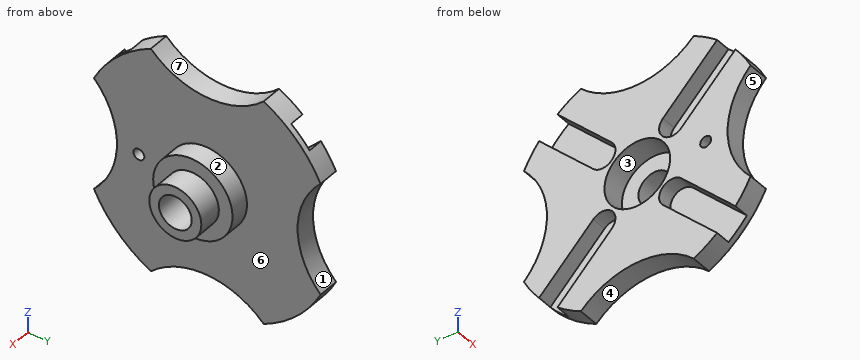
from build123d import *

# Parameters (mm, degrees)
ESQUISSE2_R             = 59
ENL_V_MAT_EXTRU_1_DEPTH = 139.666866987
ENL_V_START             = -11
ENL_V_MAT_EXTRU_2_DEPTH = 11
ESQUISSE4_R             = 4
ENL_V_MAT_EXTRU_3_DEPTH = 126.809424138


with BuildPart() as part:
    # Esquisse1 → Base-Révolution (revolve)
    with BuildSketch(Plane.XY, mode=Mode.PRIVATE) as base_r_volution_sk:
        Polygon((0, 24), (0, 92.5), (15, 92.5), (15, 29), (29, 29), (29, 19), (46, 19), (46, 12), (17, 12), (17, 24), align=None)
    revolve(base_r_volution_sk.sketch.rotate(Axis((0, 0, 0), (1, 0, 0)), 90), axis=Axis((0, 0, 0), (1, 0, 0)))

    # Esquisse2 → Enlèv. mat.-Extru.1 (cut, through all)
    with BuildSketch(Plane.ZY):
        with Locations((0, 125)):
            Circle(ESQUISSE2_R)
        with Locations((125, 0)):
            Circle(ESQUISSE2_R)
        with Locations((0, -125)):
            Circle(ESQUISSE2_R)
        with Locations((-125, 0)):
            Circle(ESQUISSE2_R)
    extrude(amount=-ENL_V_MAT_EXTRU_1_DEPTH, mode=Mode.SUBTRACT)

    # Esquisse3 → Enlèv. mat.-Extru.2 (cut)
    with BuildSketch(Plane.ZY.offset(ENL_V_START)):
        with BuildLine():
            Line((18.738329701, 32.173358544), (58.343994937, 71.77902378))
            ThreePointArc((58.343994937, 71.77902378), (65.40737726, 65.40737726), (71.77902378, 58.343994937))
            Line((71.77902378, 58.343994937), (32.173358544, 18.738329701))
            ThreePointArc((32.173358544, 18.738329701), (18.738329701, 18.738329701), (18.738329701, 32.173358544))
        make_face()
        with BuildLine():
            Line((32.173358544, -18.741271209), (71.77902378, -58.346936444))
            ThreePointArc((71.77902378, -58.346936444), (65.40737726, -65.410318767), (58.343994937, -71.781965287))
            Line((58.343994937, -71.781965287), (18.738329701, -32.176300051))
            ThreePointArc((18.738329701, -32.176300051), (18.738329701, -18.741271209), (32.173358544, -18.741271209))
        make_face()
        with BuildLine():
            Line((-18.741271209, -32.176300051), (-58.346936444, -71.781965287))
            ThreePointArc((-58.346936444, -71.781965287), (-65.410318767, -65.410318767), (-71.781965287, -58.346936444))
            Line((-71.781965287, -58.346936444), (-32.176300051, -18.741271209))
            ThreePointArc((-32.176300051, -18.741271209), (-18.741271209, -18.741271209), (-18.741271209, -32.176300051))
        make_face()
        with BuildLine():
            Line((-32.176300051, 18.738329701), (-71.781965287, 58.343994937))
            ThreePointArc((-71.781965287, 58.343994937), (-65.410318767, 65.40737726), (-58.346936444, 71.77902378))
            Line((-58.346936444, 71.77902378), (-18.741271209, 32.173358544))
            ThreePointArc((-18.741271209, 32.173358544), (-18.741271209, 18.738329701), (-32.176300051, 18.738329701))
        make_face()
    extrude(amount=ENL_V_MAT_EXTRU_2_DEPTH, mode=Mode.SUBTRACT)

    # Esquisse4 → Enlèv. mat.-Extru.3 (cut, through all)
    with BuildSketch(Plane.ZY):
        with Locations((0, -50)):
            Circle(ESQUISSE4_R)
    extrude(amount=-ENL_V_MAT_EXTRU_3_DEPTH, mode=Mode.SUBTRACT)


solid = part.part
Model file for the job. Use its own axes, mm. Face numbers are marked on the shaded views. A direction names the side the tool comes from. Coordinates: 2 decimals unless noted, no trailing zeros. Order: outer loops, then holes, each group sorted by start corner. A loop starts at its lowest first (then second) coordinate and runs counter-clockwise, first axis right, second up. Notation, with made-up numbers: (82.5, -17.5) -> (87.5, -17.5) arc R20 cw to (87.5, -7.5) -> close; hole circle Ø10 at (50.5, 87.25). An arc over 180 degrees is marked (long way). Return JSON: item names as keys, results as strings. Group by question number.
Item 1: Flat gauge pins, fed straight in: P1, Ø4, axis at x = 15, z = 59.5, coming from the +Y side; P2, Ø1, axis at x = 5, y = 55, coming from the +Z side; P3, Ø9, axis at y = -50, z = 0, coming from the +X side. Where does each tip first touch, or does it go through?
Item 2: Pull direction Y, two halves, no side cores. Call the marked faces 4, 5, 6 and 7: pulls with the +Y half, pulls with the -Y half, needs draft (parallel to the pull), parting line crosses it, or undercut.
Item 3: Tool access for the marked faces 1, 2 and 3: list every direction of +Z, -Z, +X, -X, +Y, -Y with a clear straight run to the whole face (end or side of a thin tool).
Item 4: Saw through at C-C on x = 27. Write the cut outline in (y, z), then the cut area to 3 significant figures.
Item 5: Wall check: line 1 along Y through (x, z) = (8.25, 0); line 2 along Y through (x, z) = (34.75, 0); line 3 along Z through (x, y) = (10, -17). Give the ranges that are in metal, low to high. Write a range as [from, to].
Item 6: Saw through at B-B on y = 0. Write the cut outline in (x, z).
Item 7: Saw through at A-A on z = 0. Write the cut outline in (x, y).
Item 8: Saw through at D-D on z = 62. Write the cut outline in (x, y), then the cut area to 3 significant figures.
Values found:
{
 "1": {"P1": "stops at y = 72.46", "P2": "stops at z = 74.74", "P3": "stops at x = 15"},
 "2": {"face 4": "undercut", "face 5": "pulls with the -Y half", "face 6": "needs draft", "face 7": "undercut"},
 "3": {"face 1": "+X, -X, +Y", "face 2": "+X", "face 3": "-X"},
 "4": {"outline": "circle Ø58 at (0, 0); hole circle Ø24 at (0, 0)", "area": "2,190 mm2"},
 "5": {"line 1": "y = [-66, -54], [-46, -24], [24, 66]", "line 2": "y = [-19, -12], [12, 19]", "line 3": "z = [-68.5, -29.78], [-21.13, -16.94], [16.94, 21.13], [29.78, 68.5]"},
 "6": {"outline": "(0, -66) -> (15, -66) -> (15, -29) -> (29, -29) -> (29, -19) -> (46, -19) -> (46, -12) -> (17, -12) -> (17, -24) -> (0, -24) -> close; (0, 24) -> (17, 24) -> (17, 12) -> (46, 12) -> (46, 19) -> (29, 19) -> (29, 29) -> (15, 29) -> (15, 66) -> (0, 66) -> close"},
 "7": {"outline": "(0, -66) -> (15, -66) -> (15, -54) -> (0, -54) -> close; (0, -46) -> (15, -46) -> (15, -29) -> (29, -29) -> (29, -19) -> (46, -19) -> (46, -12) -> (17, -12) -> (17, -24) -> (0, -24) -> close; (0, 24) -> (17, 24) -> (17, 12) -> (46, 12) -> (46, 19) -> (29, 19) -> (29, 29) -> (15, 29) -> (15, 66) -> (0, 66) -> close"},
 "8": {"outline": "(0, -48.57) -> (11, -48.57) -> (11, -68.65) -> (15, -68.65) -> (15, 68.65) -> (11, 68.65) -> (11, 48.56) -> (0, 48.56) -> close", "area": "1,620 mm2"}
}
